Can you work these out from the model? Positions are in its coordinate system, mm. Face numbers are marked on the shaded views. Round coordinates to 2 decimals unless told otherwise and drop trailing zeros. Write each loop counter-clockwise with the first axis right and the second up, starting at its lowest first coordinate (ties: lowest second). Pieces come first, ordered by that corner, then holes. Notation, with made-up numbers: (54, 58) -> (102, 58) arc R15 ccw to (102, 70) -> close; hole circle Ø3 at (72, -4.5). An arc over 180 degrees is marked (long way). Write item = value, one per line. Start each with the question number.
1) If I drill on line 1 (X direction, y = -4.5, z = 5.5); line 2 (X direction, y = 0.75, z = 5.5); line 3 (Z direction, x = -12, y = -5), over which ranges is the centre line in solid material (lowest first)?
2) Imagine slicing it at C-C, the plane z = 5.25. Please give me the cut outline in (x, y), then the cut area to 3 significant figures.
3) Imagine slicing it at D-D, the plane y = -2. Please give me the cut outline in (x, z).
4) Imagine slicing it at A-A, the plane y = 0. Please give me the cut outline in (x, z), then the cut area to 3 significant figures.
5) Thinking about a two-plate mould opening in Z: for the marked faces 1, 2 and 3, which applies, +Z half, -Z half, draft (parallel to the pull), parting line (faces both ways), or undercut?
6) Imagine slicing it at B-B, the plane x = -10.5. Please give me the cut outline in (y, z).
from build123d import *

# Parameters (mm, degrees)
SKETCH_1_R          = 15
EXTRUDE_1_DEPTH     = 10
CUT_EXTRUDE_1_DEPTH = 10
SKETCH_5_R          = 2
CUT_EXTRUDE_2_DEPTH = 25.779023387
SKETCH_7_W          = 30.648506912
SKETCH_7_H          = 10.688803122
CUT_EXTRUDE_4_DEPTH = 24.45207897
EXTRUDE_START       = -10
EXTRUDE_2_DEPTH     = 10


with BuildPart() as part:
    # ｽｹｯﾁ1 → ﾎﾞｽ - 押し出し1 (new body)
    with BuildSketch(Plane.XY):
        Circle(SKETCH_1_R)
    extrude(amount=EXTRUDE_1_DEPTH)

    # ｽｹｯﾁ2 → ｶｯﾄ - 押し出し1 (cut)
    with BuildSketch(Plane.XY.offset(10)):
        with BuildLine():
            Line((5.762811814, 2), (20.145888179, 2))
            Line((20.145888179, 2), (20.145888179, 26.748934653))
            Line((20.145888179, 26.748934653), (-19.854111821, 26.748934653))
            Line((-19.854111821, 26.748934653), (-19.854111821, 2))
            Line((-19.854111821, 2), (-5.762811814, 2))
            ThreePointArc((-5.762811814, 2), (0, -6.1), (5.762811814, 2))
        make_face()
    extrude(amount=-CUT_EXTRUDE_1_DEPTH, mode=Mode.SUBTRACT)

    # ｽｹｯﾁ5 → ｶｯﾄ - 押し出し2 (cut, through all)
    with BuildSketch(Plane(origin=(0, 2, 0), x_dir=(1, 0, 0), z_dir=(0, 1, 0))):
        with Locations(Location((-10.5, -5, 0), (0, 0, 270))):
            Circle(SKETCH_5_R)
        with Locations(Location((10.5, -5, 0), (0, 0, 270))):
            Circle(SKETCH_5_R)
    extrude(amount=-CUT_EXTRUDE_2_DEPTH, mode=Mode.SUBTRACT)

    # ｽｹｯﾁ7 → ｶｯﾄ - 押し出し4 (cut, through all)
    with BuildSketch(Plane.XY.offset(10)):
        with Locations((0, -13.344401561)):
            Rectangle(SKETCH_7_W, SKETCH_7_H)
    extrude(amount=-CUT_EXTRUDE_4_DEPTH, mode=Mode.SUBTRACT)

    # ｽｹｯﾁ8 → ﾎﾞｽ - 押し出し2 (add)
    with BuildSketch(Plane.XY.offset(10).offset(EXTRUDE_START)):
        with BuildLine():
            Line((-14.866068747, 2), (-15.5, 2))
            Line((-15.5, 2), (-15.5, -8))
            Line((-15.5, -8), (-12.68857754, -8))
            ThreePointArc((-12.68857754, -8), (-14.656555974, -3.191452176), (-14.866068747, 2))
        make_face()
        with BuildLine():
            ThreePointArc((14.866068747, 2), (14.656555974, -3.191452176), (12.68857754, -8))
            Line((12.68857754, -8), (15.5, -8))
            Line((15.5, -8), (15.5, 2))
            Line((15.5, 2), (14.866068747, 2))
        make_face()
    extrude(amount=EXTRUDE_2_DEPTH)


solid = part.part
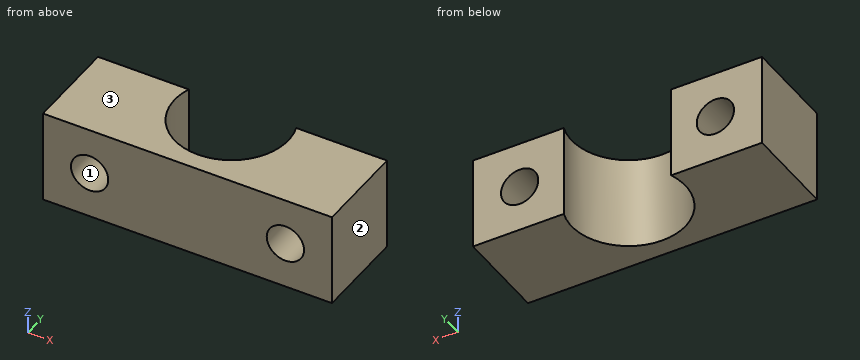
Reported:
q1.line_1 = -15.5 to -12.44, -8.56 to -4.12, 4.12 to 8.56, 12.44 to 15.5
q1.line_2 = -15.5 to -12.44, -8.56 to -6.05, 6.05 to 8.56, 12.44 to 15.5
q1.line_3 = 0 to 3.68, 6.32 to 10
q2.outline = (-15.5, -8) -> (-12.48, -8) -> (-12.48, 2) -> (-15.5, 2) -> close; (-8.52, -8) -> (8.52, -8) -> (8.52, 2) -> (5.76, 2) arc R6.1 cw (long way) to (-5.76, 2) -> (-8.52, 2) -> close; (12.48, -8) -> (15.5, -8) -> (15.5, 2) -> (12.48, 2) -> close
q2.area = 148 mm²
q3.outline = (-15.5, 0) -> (-5.76, 0) -> (-5.76, 10) -> (-15.5, 10) -> close; (5.76, 0) -> (15.5, 0) -> (15.5, 10) -> (5.76, 10) -> close; hole circle Ø4 at (-10.5, 5); hole circle Ø4 at (10.5, 5)
q4.outline = (-15.5, 0) -> (-6.1, 0) -> (-6.1, 10) -> (-15.5, 10) -> close; (6.1, 0) -> (15.5, 0) -> (15.5, 10) -> (6.1, 10) -> close; hole circle Ø4 at (-10.5, 5); hole circle Ø4 at (10.5, 5)
q4.area = 163 mm²
q5.face_1 = undercut
q5.face_2 = draft
q5.face_3 = +Z half
q6.outline = (-8, 0) -> (2, 0) -> (2, 3) -> (-8, 3) -> close; (-8, 7) -> (2, 7) -> (2, 10) -> (-8, 10) -> close
